Can you work these out from the model? Positions are in its coordinate system, mm. A direction names the side the tool comes from. Give positions to 0.01 mm unless a question says otherwise; leave off trailing zeros. Order: outer loops, then holes, each group sorted by start corner. A loop starts at its lowest first (then second) coordinate and runs counter-clockwise, first axis right, second up. Notation, with made-up numbers: (71, -28.75) -> (103, -28.75) arc R22 ccw to (103, -11.75) -> close; hole circle Ø11 at (-10.5, -4). An arc over 180 degrees is marked (long way). Answer as a JSON object with one key per item and string values.
```python
from build123d import *

# Parameters (mm, degrees)
F0_R     = 11.1
F0_R_2   = 3.6
F1_DEPTH = 6.5


with BuildPart() as f1:
    # F0 (on Top) → F1 (new body)
    with BuildSketch(Plane.XY):
        with BuildLine():
            Line((10.7278155075, -8.9952195325), (14, 0))
            Line((14, 0), (10.7278155075, 8.9952195325))
            ThreePointArc((10.7278155075, 8.9952195325), (0, 14), (-10.7278155075, 8.9952195325))
            Line((-10.7278155075, 8.9952195325), (-14, 0))
            Line((-14, 0), (-10.7278155075, -8.9952195325))
            ThreePointArc((-10.7278155075, -8.9952195325), (0, -14), (10.7278155075, -8.9952195325))
        make_face()
        Circle(F0_R, mode=Mode.SUBTRACT)
        with BuildLine():
            Line((-14, 0), (-10.7278155075, 8.9952195325))
            ThreePointArc((-10.7278155075, 8.9952195325), (-13.1565462243, 4.7859472884), (-14, 0))
        make_face()
        with BuildLine():
            ThreePointArc((-14, 0), (-13.1565462243, -4.7859472884), (-10.7278155075, -8.9952195325))
            Line((-10.7278155075, -8.9952195325), (-14, 0))
        make_face()
        with BuildLine():
            ThreePointArc((10.7278155075, -8.9952195325), (13.1565462243, -4.7859472884), (14, 0))
            Line((14, 0), (10.7278155075, -8.9952195325))
        make_face()
        with BuildLine():
            Line((10.7278155075, 8.9952195325), (14, 0))
            ThreePointArc((14, 0), (13.1565462243, 4.7859472884), (10.7278155075, 8.9952195325))
        make_face()
        with BuildLine():
            ThreePointArc((-6.3985424017, 20.896370611), (0, 18.8439208418), (6.3985424017, 20.896370611))
            Line((6.3985424017, 20.896370611), (2.8967563366, 30.5227637692))
            ThreePointArc((2.8967563366, 30.5227637692), (1.1947786179, 32.4754527121), (1.2443241353, 35.0652919937))
            Line((1.2443241353, 35.0652919937), (0, 38.4859330952))
            Line((0, 38.4859330952), (-1.2735454835, 34.9849626471))
            ThreePointArc((-1.2735454835, 34.9849626471), (-1.0979323396, 34.3562319579), (-1.0387459151, 33.706124872))
            ThreePointArc((-1.0387459151, 33.706124872), (-1.5334959699, 31.8847455108), (-2.8817585693, 30.5639925599))
            Line((-2.8817585693, 30.5639925599), (-6.3985424017, 20.896370611))
        make_face()
        with Locations((0, 26.1885132641)):
            Circle(F0_R_2, mode=Mode.SUBTRACT)
        with BuildLine():
            Line((2.8967563366, 30.5227637692), (6.3985424017, 20.896370611))
            ThreePointArc((6.3985424017, 20.896370611), (9.7822279267, 24.8132134571), (11, 29.8439208418))
            ThreePointArc((11, 29.8439208418), (-5.0307073847, 39.6261487685), (-6.3985424017, 20.896370611))
            Line((-6.3985424017, 20.896370611), (-2.8817585693, 30.5639925599))
            ThreePointArc((-2.8817585693, 30.5639925599), (-8.0218578014, 34.9367970319), (-1.2735454835, 34.9849626471))
            Line((-1.2735454835, 34.9849626471), (0, 38.4859330952))
            Line((0, 38.4859330952), (1.2443241353, 35.0652919937))
            ThreePointArc((1.2443241353, 35.0652919937), (5.2704080391, 37.2388885867), (8.1778905042, 33.706124872))
            ThreePointArc((8.1778905042, 33.706124872), (6.4363733527, 30.6229379653), (2.8967563366, 30.5227637692))
        make_face()
        with BuildLine():
            ThreePointArc((-10.7278155075, 8.9952195325), (0, 14), (10.7278155075, 8.9952195325))
            Line((10.7278155075, 8.9952195325), (6.3985424017, 20.896370611))
            ThreePointArc((6.3985424017, 20.896370611), (0, 18.8439208418), (-6.3985424017, 20.896370611))
            Line((-6.3985424017, 20.896370611), (-10.7278155075, 8.9952195325))
        make_face()
        with BuildLine():
            Line((3.2549400142, -29.5381185512), (6.3985424017, -20.896370611))
            ThreePointArc((6.3985424017, -20.896370611), (0, -18.8439208418), (-6.3985424017, -20.896370611))
            Line((-6.3985424017, -20.896370611), (-3.2654211785, -29.5093058806))
            ThreePointArc((-3.2654211785, -29.5093058806), (-1.6042656478, -30.8323566496), (-0.9778905042, -32.8615326434))
            ThreePointArc((-0.9778905042, -32.8615326434), (-1.0897360598, -33.7519137821), (-1.4183230442, -34.5869698246))
            Line((-1.4183230442, -34.5869698246), (0, -38.4859330952))
            Line((0, -38.4859330952), (1.4430277894, -34.5190565983))
            ThreePointArc((1.4430277894, -34.5190565983), (1.2556340289, -31.6308604836), (3.2549400142, -29.5381185512))
        make_face()
        with Locations((0, -25.3439210355)):
            Circle(F0_R_2, mode=Mode.SUBTRACT)
        with BuildLine():
            Line((6.3985424017, -20.896370611), (10.7278155075, -8.9952195325))
            ThreePointArc((10.7278155075, -8.9952195325), (0, -14), (-10.7278155075, -8.9952195325))
            Line((-10.7278155075, -8.9952195325), (-6.3985424017, -20.896370611))
            ThreePointArc((-6.3985424017, -20.896370611), (0, -18.8439208418), (6.3985424017, -20.896370611))
        make_face()
        with BuildLine():
            ThreePointArc((11, -29.8439208418), (9.7822279267, -24.8132134571), (6.3985424017, -20.896370611))
            Line((6.3985424017, -20.896370611), (3.2549400142, -29.5381185512))
            ThreePointArc((3.2549400142, -29.5381185512), (6.6360314176, -29.8663948133), (8.2387459151, -32.8615326434))
            ThreePointArc((8.2387459151, -32.8615326434), (5.4918035765, -36.3590021038), (1.4430277894, -34.5190565983))
            Line((1.4430277894, -34.5190565983), (0, -38.4859330952))
            Line((0, -38.4859330952), (-1.4183230442, -34.5869698246))
            ThreePointArc((-1.4183230442, -34.5869698246), (-7.9610023904, -34.0922048033), (-3.2654211785, -29.5093058806))
            Line((-3.2654211785, -29.5093058806), (-6.3985424017, -20.896370611))
            ThreePointArc((-6.3985424017, -20.896370611), (-5.0307073847, -39.6261487685), (11, -29.8439208418))
        make_face()
    extrude(amount=F1_DEPTH)


solid = f1.part
```
1. Please list where these lines run through material, in increasing order: L1, parallel to Y at x = 0, z = 3.75; L2, parallel to X at y = 0.5, z = 2.75; L3, parallel to Y at x = -2.5, z = 3.
Worked answers:
{"L1": "-40.84 to -28.94, -21.74 to -11.1, 11.1 to 22.59, 29.79 to 40.84", "L2": "-13.99 to -11.09, 11.09 to 13.99", "L3": "-40.56 to -35.8, -29.92 to -27.93, -22.75 to -10.81, 10.81 to 23.6, 28.78 to 30.81, 36.6 to 40.56"}
2. For faces 1 (the face through (-0.469, 29.758, 3.204)), 2 (the face through (-8.533, 15.029, 3.204)), 3 (the face through (8.593, 14.862, 3.204)), which set-ups out of +Z, -Z, +X, -X, +Y, -Y let a thin tool reach every point of the face, with its end or its side?
Worked answers:
{"face 1": "+Z, -Z", "face 2": "+Z, -Z, -X", "face 3": "+Z, -Z, +X"}
3. If we mould it in two halves opening along Y, with no side actions, what happens to faces 4 (the face through (-8.593, -14.862, 3.204)), 5 (the face through (-6, 10, 6.5))? For each: +Y half, -Y half, draft (parallel to the pull), parting line (faces both ways), or undercut.
Worked answers:
{"face 4": "undercut", "face 5": "draft"}
4. If we section it at C-C on z = 2.25: Please give me the cut outline in (x, y), then the cut area to 3 significant figures.
Worked answers:
{"outline": "(-10.73, -9) -> (-6.4, -20.9) arc R11 ccw (long way) to (6.4, -20.9) -> (10.73, -9) arc R14 ccw to (10.73, 9) -> (6.4, 20.9) arc R11 ccw (long way) to (-6.4, 20.9) -> (-10.73, 9) arc R14 ccw to start; hole circle Ø22.2 at (0, 0); hole circle Ø7.2 at (-4.64, 33.71); hole circle Ø7.2 at (-4.58, -32.86); hole circle Ø7.2 at (0, -25.34); hole circle Ø7.2 at (0, 26.19); hole circle Ø7.2 at (4.58, 33.71); hole circle Ø7.2 at (4.64, -32.86)", "area": "967 mm²"}
5. If we section it at A-A on x = 0: Please give me the cut outline in (y, z), then the cut area to 3 significant figures.
Worked answers:
{"outline": "(-40.84, 0) -> (-28.94, 0) -> (-28.94, 6.5) -> (-40.84, 6.5) -> close; (-21.74, 0) -> (-11.1, 0) -> (-11.1, 6.5) -> (-21.74, 6.5) -> close; (11.1, 0) -> (22.59, 0) -> (22.59, 6.5) -> (11.1, 6.5) -> close; (29.79, 0) -> (40.84, 0) -> (40.84, 6.5) -> (29.79, 6.5) -> close", "area": "293 mm²"}
6. Will these pins go through, and if not, where does the flat tip stop? pin 1 Ø3 at (y, z) = (-28, 2) entering from +X; pin 2 Ø11.5 at (x, y) = (4.64, -32.86) entering from -Z; pin 3 Ø3 at (x, z) = (-4, 1) entering from -Y; pin 4 Ø6.5 at (x, y) = (-4.58, -32.86) entering from -Z.
Worked answers:
{"pin 1": "x = 10.99", "pin 2": "z = 0", "pin 3": "y = -40.56", "pin 4": "through"}
7. If we section it at B-B on y = 28.5: Please give me the cut outline in (x, z).
Worked answers:
{"outline": "(-10.92, 0) -> (-2.76, 0) -> (-2.76, 6.5) -> (-10.92, 6.5) -> close; (2.76, 0) -> (10.92, 0) -> (10.92, 6.5) -> (2.76, 6.5) -> close"}
8. If we section it at D-D on x = -9.5: Please give me the cut outline in (y, z), then the cut area to 3 significant figures.
Worked answers:
{"outline": "(-35.39, 0) -> (-24.3, 0) -> (-24.3, 6.5) -> (-35.39, 6.5) -> close; (-12.37, 0) -> (-5.74, 0) -> (-5.74, 6.5) -> (-12.37, 6.5) -> close; (5.74, 0) -> (12.37, 0) -> (12.37, 6.5) -> (5.74, 6.5) -> close; (24.3, 0) -> (35.39, 0) -> (35.39, 6.5) -> (24.3, 6.5) -> close", "area": "230 mm²"}
